from build123d import *

# Parameters (mm, degrees)
SKETCH1_R           = 21
BOSS_EXTRUDE1_DEPTH = 17.9451
BOSS_EXTRUDE2_START = -17.9451
SKETCH2_R           = 11
BOSS_EXTRUDE2_DEPTH = 20.0025
SKETCH3_R           = 4
BOSS_EXTRUDE4_DEPTH = 19.9426
CUT_EXTRUDE1_DEPTH  = 15
SKETCH5_R           = 1.5
CUT_EXTRUDE2_DEPTH  = 4
SKETCH6_R           = 2.5
BOSS_EXTRUDE5_DEPTH = 19.9426
CUT_EXTRUDE3_DEPTH  = 16.9426
SKETCH9_R           = 5
BOSS_EXTRUDE6_DEPTH = 20.701


with BuildPart() as part:
    # Sketch1 → Boss-Extrude1 (new body, symmetric)
    with BuildSketch(Plane(origin=(0, 0, 0), x_dir=(1, 0, 0), z_dir=(0, 1, 0))):
        Circle(SKETCH1_R)
    extrude(amount=BOSS_EXTRUDE1_DEPTH, both=True)

    # Sketch2 → Boss-Extrude2 (add, symmetric)
    with BuildSketch(Plane(origin=(0, 17.9451, 0), x_dir=(1, 0, 0), z_dir=(0, 1, 0)).offset(BOSS_EXTRUDE2_START)):
        Circle(SKETCH2_R)
    extrude(amount=BOSS_EXTRUDE2_DEPTH, both=True)

    # Sketch3 → Boss-Extrude4 (add)
    with BuildSketch(Plane(origin=(0, 20.0025, 0), x_dir=(1, 0, 0), z_dir=(0, 1, 0))):
        Circle(SKETCH3_R)
    extrude(amount=BOSS_EXTRUDE4_DEPTH)

    # Sketch4 → Cut-Extrude1 (cut)
    with BuildSketch(Plane(origin=(0, 39.9451, 0), x_dir=(1, 0, 0), z_dir=(0, 1, 0))):
        with BuildLine():
            Line((-2.645751311, 3), (2.645751311, 3))
            ThreePointArc((2.645751311, 3), (0, 4), (-2.645751311, 3))
        make_face()
    extrude(amount=-CUT_EXTRUDE1_DEPTH, mode=Mode.SUBTRACT)

    # Sketch5 → Cut-Extrude2 (cut)
    with BuildSketch(Plane(origin=(0, 17.9451, 0), x_dir=(1, 0, 0), z_dir=(0, 1, 0))):
        with Locations((0, 14)):
            Circle(SKETCH5_R)
        with Locations((-14, 0)):
            Circle(SKETCH5_R)
        with Locations((0, -14)):
            Circle(SKETCH5_R)
        with Locations((14, 0)):
            Circle(SKETCH5_R)
    extrude(amount=-CUT_EXTRUDE2_DEPTH, mode=Mode.SUBTRACT)

    # Sketch6 → Boss-Extrude5 (add)
    with BuildSketch(Plane.XZ.offset(20.0025)):
        Circle(SKETCH6_R)
    extrude(amount=BOSS_EXTRUDE5_DEPTH)

    # Sketch7 → Cut-Extrude3 (cut)
    with BuildSketch(Plane.XZ.offset(39.9451)):
        with BuildLine():
            Line((-2, -1.5), (2, -1.5))
            ThreePointArc((2, -1.5), (0, -2.5), (-2, -1.5))
        make_face()
    extrude(amount=-CUT_EXTRUDE3_DEPTH, mode=Mode.SUBTRACT)

    # Sketch9 → Boss-Extrude6 (add, symmetric)
    with BuildSketch(Plane(origin=(0, 0, 0), x_dir=(1, 0, 0), z_dir=(0, 1, 0))):
        Circle(SKETCH9_R)
    extrude(amount=BOSS_EXTRUDE6_DEPTH, both=True)


solid = part.part
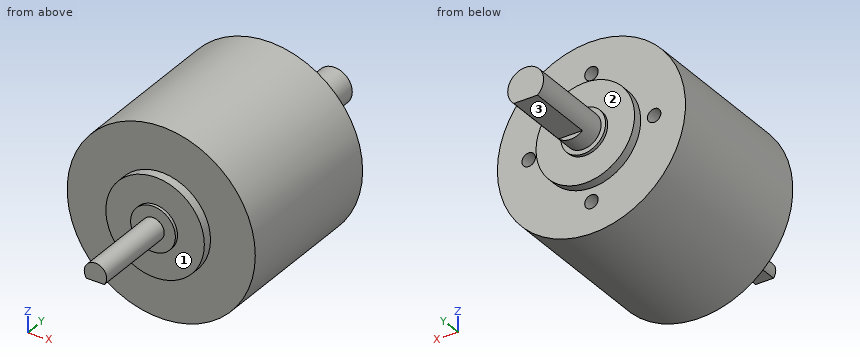
The listing builds one solid part. Answer for the finished solid, in the listing's coordinates (mm). Face numbers are marked on the shaded views. A direction names the side the tool comes from. Give positions to 0.01 mm unless a question says otherwise; leave off trailing zeros. Order: outer loops, then holes, each group sorted by start corner. A loop starts at its lowest first (then second) coordinate and runs counter-clockwise, first axis right, second up. Notation, with made-up numbers: (74, -27.75) - (128, -27.75) arc R10 ccw to (128, -23.75) - close; hole circle Ø9 at (-26.5, 28.5). An arc over 180 degrees is marked (long way). Answer as CSV lines item,"result".
Q1. Which of the six approach directions +Z, -Z, +X, -X, +Y, -Y give full straight-line access (tool end or side, diameter ignored) to the marked faces 1, 2 and 3?
Answer key:
face 1,"-Y"
face 2,"+Y"
face 3,"-Z, +X, -X, +Y"
Q2. Each of these flat-tipped pins is pushed along its axis until it touches: pin 1 Ø1.8 at (x, z) = (-14, 0) entering from +Y; pin 2 Ø2 at (y, z) = (31.5, 4) entering from +X; pin 3 Ø1 at (y, z) = (6, 6.5) entering from -X. Where does it stop, or does it pass through?
Answer key:
pin 1,"stops at y = 13.95"
pin 2,"stops at x = 2.65"
pin 3,"stops at x = -20.12"
Q3. Straight lines are drawn through the part: L1, parallel to Z at x = 0, y = 14; L2, parallel to Y at x = 5, z = -13. For each, find the intervals that lie inside material, in ascending order.
Answer key:
L1,"z = -21 to -15.5, -12.5 to 12.5, 15.5 to 21"
L2,"y = -17.95 to 17.95"
Q4. A cutting plane is placed at D-D, the plane y = 31.5. Determine the outline of the cut face in (x, z).
Answer key:
outline,"(-2.65, -3) - (2.65, -3) arc R4 ccw (long way) to start"
Q5. A cutting plane is placed at A-A, the plane y = 16. Determine the outline of the cut face in (x, z), and give its area (3 significant figures).
Answer key:
outline,"circle Ø42 at (0, 0); hole circle Ø3 at (-14, 0); hole circle Ø3 at (0, -14); hole circle Ø3 at (0, 14); hole circle Ø3 at (14, 0)"
area,"1,360 mm^2"
Q6. A cutting plane is placed at B-B, the plane x = 14. Determine the outline of the cut face in (y, z).
Answer key:
outline,"(-17.95, -15.65) - (17.95, -15.65) - (17.95, -1.5) - (13.95, -1.5) - (13.95, 1.5) - (17.95, 1.5) - (17.95, 15.65) - (-17.95, 15.65) - close"
Q7. A cutting plane is placed at C-C, the plane z = -8.5. Determine the outline of the cut face in (x, y), and give its area (3 significant figures).
Answer key:
outline,"(-19.2, -17.95) - (-6.98, -17.95) - (-6.98, -20) - (6.98, -20) - (6.98, -17.95) - (19.2, -17.95) - (19.2, 17.95) - (6.98, 17.95) - (6.98, 20) - (-6.98, 20) - (-6.98, 17.95) - (-19.2, 17.95) - close"
area,"1,440 mm^2"
